The listing builds one solid part. Answer for the finished solid, in the listing's coordinates (mm). Face numbers are marked on the shaded views. A direction names the side the tool comes from. Coordinates: 2 decimals unless noted, no trailing zeros. Write each loop counter-clockwise with the first axis right and the second up, starting at its lowest first coordinate (ties: lowest second). Pieces come first, ordered by that corner, then holes.
from build123d import *


with BuildPart() as part:
    # Sketch1 → Revolve1 (revolve)
    with BuildSketch(Plane.XY):
        with BuildLine():
            Line((-35, 0), (-47.5, 0))
            Line((-47.5, 0), (-47.5, 3.175))
            ThreePointArc((-47.5, 3.175), (-45.9125, 4.7625), (-47.5, 6.35))
            Line((-47.5, 6.35), (-47.5, 12))
            Line((-47.5, 12), (-45, 12))
            Line((-45, 12), (-45, 10))
            Line((-45, 10), (-37.5, 10))
            Line((-37.5, 10), (-37.5, 12))
            Line((-37.5, 12), (0, 12))
            Line((0, 12), (0, 0))
            Line((0, 0), (-28.65, 0))
            Line((-28.65, 0), (-28.65, 3.8))
            Line((-28.65, 3.8), (-35, 3.8))
            Line((-35, 3.8), (-35, 0))
        make_face()
    revolve(axis=Axis((0, 0, 0), (0, -1, 0)))


solid = part.part
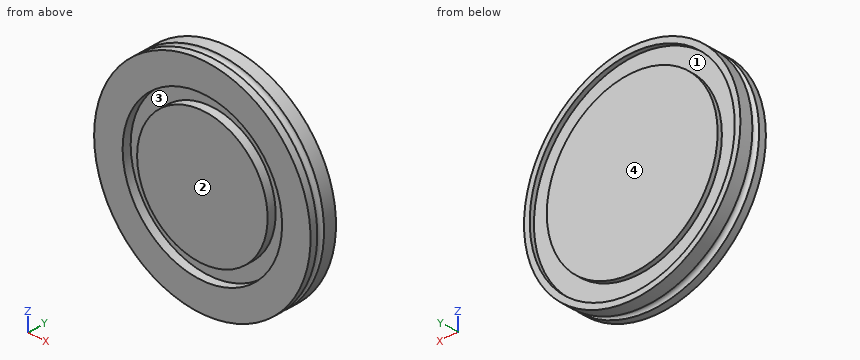
Q1. Determine the mould class of the marked faces 3 and 4 for opening direction Z: released by +Z, released by -Z, zero draft, split by the parting line, or undercut.
Answers below:
face 3: undercut
face 4: zero draft
Q2. Find the intervals of material crossed by probe 1 along X at (y, z) = (2.05, 0); probe 2 along X at (y, z) = (11.4, 0), in increasing order.
Answers below:
probe 1: x = -47.5 to -35, -28.65 to 28.65, 35 to 47.5
probe 2: x = -47.5 to -45, -37.5 to 37.5, 45 to 47.5
Q3. Given pin 1 (1.5 mm diameter, centred on x = 5, y = 5, fed in from -Z); pin 2 (6 mm diameter, centred on x = -8, y = 4.5, fed in from -Z); pin 3 (1 mm diameter, centred on y = 7.5, z = -15, fed in from +X); pin 4 (10 mm diameter, centred on x = -27, z = 10, fed in from -Y), each flat-ended and moving along its own axis, determine where each tip first touches the part or whether it passes through.
Answers below:
pin 1: stops at z = -45.99
pin 2: stops at z = -47.2
pin 3: stops at x = 45.23
pin 4: stops at y = 0
Q4. Which of the six approach directions +Z, -Z, +X, -X, +Y, -Y give full straight-line access (tool end or side, diameter ignored) to the marked faces 1 and 2?
Answers below:
face 1: +Y
face 2: +Z, -Z, +X, -X, -Y
Q5. The part is cut by section C-C, the plane y = 5. Write down the section's boundary in (x, z).
Answers below:
outline: circle Ø91.86 at (0, 0)
